from build123d import *

# Parameters (mm, degrees)
SKETCH_1_R      = 1.35
SKETCH_1_R_2    = 5.1
EXTRUDE_1_DEPTH = 3


with BuildPart() as part:
    # 草图1 → 凸台-拉伸1 (new body)
    with BuildSketch(Plane(origin=(0, 0, 0), x_dir=(0, 0, -1), z_dir=(1, 0, 0))):
        with BuildLine():
            Line((-14, 0), (-14, 108))
            Line((-14, 108), (14, 108))
            Line((14, 108), (14, 0))
            ThreePointArc((14, 0), (0, -14), (-14, 0))
        make_face()
        with Locations((0, -11)):
            Circle(SKETCH_1_R, mode=Mode.SUBTRACT)
        with Locations((-7.778174593, -7.778174593)):
            Circle(SKETCH_1_R, mode=Mode.SUBTRACT)
        with Locations((-11, 0)):
            Circle(SKETCH_1_R, mode=Mode.SUBTRACT)
        with Locations((-7.778174593, 7.778174593)):
            Circle(SKETCH_1_R, mode=Mode.SUBTRACT)
        with Locations((0, 11)):
            Circle(SKETCH_1_R, mode=Mode.SUBTRACT)
        with Locations((7.778174593, 7.778174593)):
            Circle(SKETCH_1_R, mode=Mode.SUBTRACT)
        with Locations((11, 0)):
            Circle(SKETCH_1_R, mode=Mode.SUBTRACT)
        with Locations((7.778174593, -7.778174593)):
            Circle(SKETCH_1_R, mode=Mode.SUBTRACT)
        Circle(SKETCH_1_R_2, mode=Mode.SUBTRACT)
        with Locations((-11, 105)):
            Circle(SKETCH_1_R, mode=Mode.SUBTRACT)
        with Locations(Location((11, 105, 0), (0, 0, 180))):
            Circle(SKETCH_1_R, mode=Mode.SUBTRACT)
    extrude(amount=EXTRUDE_1_DEPTH)


solid = part.part
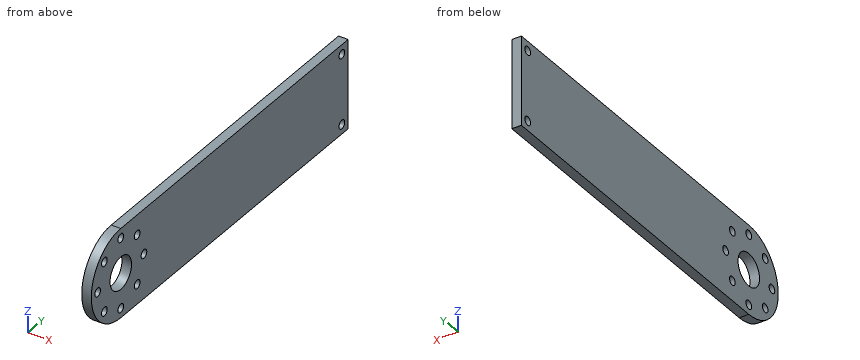
CAD build for the part. Positions are in the model's coordinates, mm. Coordinates: 2 decimals unless noted, no trailing zeros. Loops run counter-clockwise (first coordinate to the right, second up) from the corner with the lowest first, then second, coordinate; pieces in that order, holes last. Notation, with made-up numbers: (65.5, 73.5) - (77.5, 73.5) arc R12 cw to (77.5, 86.5) - close; hole circle Ø9 at (5, 55). An arc over 180 degrees is marked (long way). Write item = value, one per line. Start each with the question number.
Q1. Cut at D-D, the plane z = 2.5. List the corners of the cut face in (x, y).
Q2. Cut at C-C, the plane x = 1.65. Give the number of separate pieces and of enclosed holes in the cut face, then the cut area to 3 significant figures.
Q3. Cut at B-B, the plane y = -11. List the corners of the cut face in (x, z).
Q4. Drill centre lines: L1, parallel to Z at x = 1.1, y = 105; L2, parallel to Y at x = 1.75, z = 0; L3, parallel to Y at x = 1.05, z = -10.5. Where is each one in solid material? Low to high.
Q5. Cut at A-A, the plane z = 11. List the corners of the cut face in (x, y).
Computed:
q1.outline = (0, -13.77) - (3, -13.77) - (3, -4.45) - (0, -4.45) - close; (0, 4.45) - (3, 4.45) - (3, 108) - (0, 108) - close
q2.separate_pieces = 1
q2.enclosed_holes = 11
q2.area = 3,190 mm²
q3.outline = (0, -8.66) - (3, -8.66) - (3, -1.35) - (0, -1.35) - close; (0, 1.35) - (3, 1.35) - (3, 8.66) - (0, 8.66) - close
q4.L1 = -14 to -12.35, -9.65 to 9.65, 12.35 to 14
q4.L2 = -14 to -12.35, -9.65 to -5.1, 5.1 to 9.65, 12.35 to 108
q4.L3 = -9.26 to -1.25, 1.25 to 103.75, 106.25 to 108
q5.outline = (0, -8.66) - (3, -8.66) - (3, -1.35) - (0, -1.35) - close; (0, 1.35) - (3, 1.35) - (3, 103.65) - (0, 103.65) - close; (0, 106.35) - (3, 106.35) - (3, 108) - (0, 108) - close
